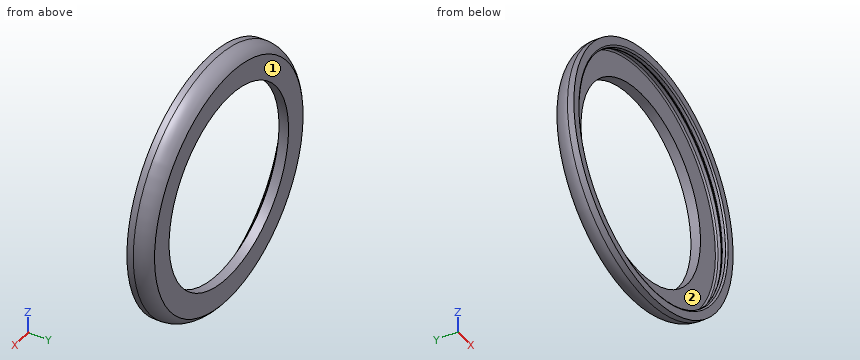
```python
from build123d import *

# Parameters (mm, degrees)
REDONDEO1_R = 0.25


with BuildPart() as part:
    # Croquis1 → Revolución1 (revolve)
    with BuildSketch(Plane.XY, mode=Mode.PRIVATE) as revoluci_n1_sk:
        with BuildLine():
            Line((20, 0), (20, 1))
            ThreePointArc((20, 1), (19.643382037, 2.418637165), (18.658312395, 3.5))
            Line((18.658312395, 3.5), (15, 3.5))
            Line((15, 3.5), (15, 2))
            Line((15, 2), (19, 2))
            Line((19, 2), (19, 1))
            Line((19, 1), (18.5, 1))
            Line((18.5, 1), (18.5, 0))
            Line((18.5, 0), (20, 0))
        make_face()
    revolve(revoluci_n1_sk.sketch.rotate(Axis((0, 0, 0), (0, 1, 0)), 90), axis=Axis((0, 0, 0), (0, 1, 0)))

    # Redondeo1
    redondeo1_edges = [part.edges().sort_by_distance(p)[0] for p in [
        (0, 0, 18.5),
        (0, 1, 18.5),
        (0, 1, 19),
        (0, 2, 19),
    ]]
    fillet(redondeo1_edges, radius=REDONDEO1_R - 0.0001)  # a hair under: the kernel refuses the full size


solid = part.part
```
The listing builds one solid part. Answer for the finished solid, in the listing's coordinates (mm). Face numbers are marked on the shaded views. Give positions to 0.01 mm unless a question says otherwise; leave off trailing zeros. Order: outer loops, then holes, each group sorted by start corner. A loop starts at its lowest first (then second) coordinate and runs counter-clockwise, first axis right, second up. Notation, with made-up numbers: (-32, 38) - (27, 38) arc R24 cw to (27, 59) - close; hole circle Ø9 at (-8.75, 15.5). An arc over 180 degrees is marked (long way). Use one line per item in the form item = value. Start each with the question number.
(1) Flat-ended cylindrical pins translate along their axes: pin 1 Ø4 at (x, z) = (14, 6) entering from -Y; pin 2 Ø1 at (x, y) = (-12, 1) entering from +Z. Find the tip coordinate at first contact, or state that the pin passes through.
(2) The mould has two halves that part along Z. Classify the marked faces 1 and 2: released by +Z, released by -Z, zero draft, split by the parting line, or undercut.
(3) Consider line 1 (X direction, y = 0.65, z = 0); line 2 (Y direction, x = 8, z = -16); line 3 (X direction, y = 1.6, z = 0). Determine where each line is inside the solid, lowest interval first. Write a range as from..to.
(4) A cutting plane is placed at C-C, the plane y = 3. Write down the section's boundary in (x, z).
Ans:
q1.pin_1 = 2
q1.pin_2 = 16.36
q2.face_1 = zero draft
q2.face_2 = undercut
q3.line_1 = -20..-18.5, 18.5..20
q3.line_2 = 2..3.5
q3.line_3 = -19.94..-19, 19..19.94
q4.outline = circle Ø38.47 at (0, 0); hole circle Ø30 at (0, 0)
